from build123d import *

# Parameters (mm, degrees)
F1_DEPTH = 12.5
F3_DEPTH = 25
F4_R     = 9.05
F5_DEPTH = 55
F6_R     = 9.05
F7_DEPTH = 52.5
F9_DEPTH = 3


with BuildPart() as f1:
    # F0 (on Top) → F1 (new body, symmetric)
    with BuildSketch(Plane.XY):
        with BuildLine():
            ThreePointArc((50, 0), (0, -50), (-50, 0))
            Line((-50, 0), (-55, 0))
            ThreePointArc((-55, 0), (0, -55), (55, 0))
            Line((55, 0), (50, 0))
        make_face()
    extrude(amount=F1_DEPTH, both=True)

    # F2 (on face) → F3 (join)
    with BuildSketch(Plane.XY.offset(12.5)):
        with BuildLine():
            ThreePointArc((55, 0), (0, -55), (-55, 0))
            Line((-55, 0), (-55, -57.5))
            Line((-55, -57.5), (0, -57.5))
            Line((0, -57.5), (55, -57.5))
            Line((55, -57.5), (55, 0))
        make_face()
    extrude(amount=-F3_DEPTH)

    # F4 (on Front) → F5 (cut)
    with BuildSketch(Plane.XZ):
        Circle(F4_R)
    extrude(amount=F5_DEPTH, mode=Mode.SUBTRACT)

    # F6 (on Right) → F7 (cut, symmetric)
    with BuildSketch(Plane.YZ):
        with Locations((-11, 0)):
            Circle(F6_R)
    extrude(amount=F7_DEPTH, both=True, mode=Mode.SUBTRACT)

    # F8 (on face) → F9 (join)
    with BuildSketch(Plane.XZ.offset(57.5)):
        with BuildLine():
            Line((55, -1.825145), (56.187007, -1.825145))
            ThreePointArc((56.187007, -1.825145), (73.996764, 0.241309), (56.101841, 1.350101))
            Line((56.101841, 1.350101), (55, 1.350101))
            Line((55, 1.350101), (55, -1.825145))
        make_face()
        with BuildLine():
            Line((-55, 0.589209), (-56.019308, 0.589209))
            ThreePointArc((-56.019308, 0.589209), (-73.999691, -0.074534), (-56.010781, -0.440385))
            Line((-56.010781, -0.440385), (-55, -0.440385))
            Line((-55, -0.440385), (-55, 0.589209))
        make_face()
        with BuildLine():
            Line((26.665892, -12.5), (26.665892, -13.538735))
            ThreePointArc((26.665892, -13.538735), (27.491135, -31.499996), (28.35176, -13.540396))
            Line((28.35176, -13.540396), (28.35176, -12.5))
            Line((28.35176, -12.5), (26.665892, -12.5))
        make_face()
        with BuildLine():
            Line((-28.294771, -12.5), (-28.294771, -13.535161))
            ThreePointArc((-28.294771, -13.535161), (-27.521055, -31.499975), (-26.663293, -13.538978))
            Line((-26.663293, -13.538978), (-26.663293, -12.5))
            Line((-26.663293, -12.5), (-28.294771, -12.5))
        make_face()
        with BuildLine():
            Line((-26.327094, 12.5), (-26.327094, 13.576756))
            ThreePointArc((-26.327094, 13.576756), (-27.667739, 31.498437), (-28.339533, 13.539242))
            Line((-28.339533, 13.539242), (-28.339533, 12.5))
            Line((-28.339533, 12.5), (-26.327094, 12.5))
        make_face()
        with BuildLine():
            Line((28.639116, 12.5), (28.639116, 13.572379))
            ThreePointArc((28.639116, 13.572379), (27.368028, 31.499032), (26.623167, 13.542815))
            Line((26.623167, 13.542815), (26.623167, 12.5))
            Line((26.623167, 12.5), (28.639116, 12.5))
        make_face()
    extrude(amount=-F9_DEPTH)


solid = f1.part
Verification items for the finished model (mm, model axes). A direction names the side the tool comes from. Give positions to 0.01 mm unless a question says otherwise; leave off trailing zeros. Loops run counter-clockwise (first coordinate to the right, second up) from the corner with the lowest first, then second, coordinate; pieces in that order, holes last. Notation, with made-up numbers: (39.25, -29.75) - (92.25, -29.75) arc R33 cw to (92.25, 5.25) - close; hole circle Ø9 at (67, 68.5). An arc over 180 degrees is marked (long way). Write each question's results on one line, items separated by ' | '.
1) Sectioned sample at B-B on y = -6. Record the boundary of the cut face in (x, z), plus the area to 3 significant figures.
Solution:
outline: (-55, -12.5) - (-49.64, -12.5) - (-49.64, -7.54) - (-52.5, -7.54) - (-52.5, 7.54) - (-49.64, 7.54) - (-49.64, 12.5) - (-55, 12.5) - close; (49.64, -12.5) - (55, -12.5) - (55, 12.5) - (49.64, 12.5) - (49.64, 7.54) - (52.5, 7.54) - (52.5, -7.54) - (49.64, -7.54) - close | area: 182 mm2
2) Material ranges on L1, parallel to X at y = -53, z = 0; L2, parallel to Z at x = 0, y = -52; L3, parallel to Y at x = -47.75, z = 0, recorded low to high. Write a range as from..to.
Solution:
L1: -55..-9.05, 9.05..55 | L2: -12.5..-9.05, 9.05..12.5 | L3: -57.5..-20.05
3) Sectioned sample at C-C on x = 0. Record the boundary of the cut face in (y, z), plus the area to 3 significant figures.
Solution:
outline: (-57.5, -12.5) - (-50, -12.5) - (-50, -9.05) - (-55, -9.05) - (-55, 9.05) - (-50, 9.05) - (-50, 12.5) - (-57.5, 12.5) - close | area: 97.0 mm2
4) Tool access check on faces 1 (the flat face through (-28, -54.5, 22)), 2 (the flat face through (-65, -54.5, 0)), 3 (the flat face through (0, -55, 0)), 4 (the flat face through (64, -54.5, 0)), 5 (the cylindrical face through (-49.85, -20.04, 0.4)). Record the directions out of +Z, -Z, +X, -X, +Y, -Y that give a thin tool (end or side, any length) a straight path to the whole face; none if there is none.
Solution:
face 1: +Z, +X, -X, +Y | face 2: +Z, -Z, -X, +Y | face 3: +Y | face 4: +Z, -Z, +X, +Y | face 5: none
5) Mould release check, pull along X, two halves, no side actions. Record for faces 6 (the flat face through (27, -54.5, -22)), 7 (the cylindrical face through (8.63, -52.05, 2.72)): pulls with the +X half, pulls with the -X half, needs draft (parallel to the pull), parting line crosses it, or undercut.
Solution:
face 6: needs draft | face 7: undercut
6) Depth check by flat-ended pin: P1, Ø20, axis at x = -31, z = 20, coming from the +Y side; P2, Ø1.1, axis at y = -56.5, z = -13, coming from the -X side; P3, Ø2, axis at x = -29.5, y = -42, coming from the +Z side. Enter the tip coordinate at first touch or a pass-through.
Solution:
P1: y = -32.94 | P2: x = -55 | P3: z = 12.5
7) Sectioned sample at A-A on z = -22.5. Record the boundary of the cut face in (x, y).
Solution:
outline: (-36.5, -57.5) - (-18.5, -57.5) - (-18.5, -54.5) - (-36.5, -54.5) - close; (18.5, -57.5) - (36.5, -57.5) - (36.5, -54.5) - (18.5, -54.5) - close
8) Sectioned sample at D-D on z = 5.5. Record the boundary of the cut face in (x, y).
Solution:
outline: (-72.12, -57.5) - (-57.88, -57.5) - (-57.88, -54.5) - (-72.12, -54.5) - close; (-55, -57.5) - (55, -57.5) - (55, 0) - (50, 0) arc R50 cw to (49.85, -3.81) - (52.5, -3.81) - (52.5, -18.19) - (46.58, -18.19) arc R50 cw to (7.19, -49.48) - (7.19, -55) - (-7.19, -55) - (-7.19, -49.48) arc R50 cw to (-46.58, -18.19) - (-52.5, -18.19) - (-52.5, -3.81) - (-49.85, -3.81) arc R50 cw to (-50, 0) - (-55, 0) - close; (57.88, -57.5) - (72.12, -57.5) - (72.12, -54.5) - (57.88, -54.5) - close
